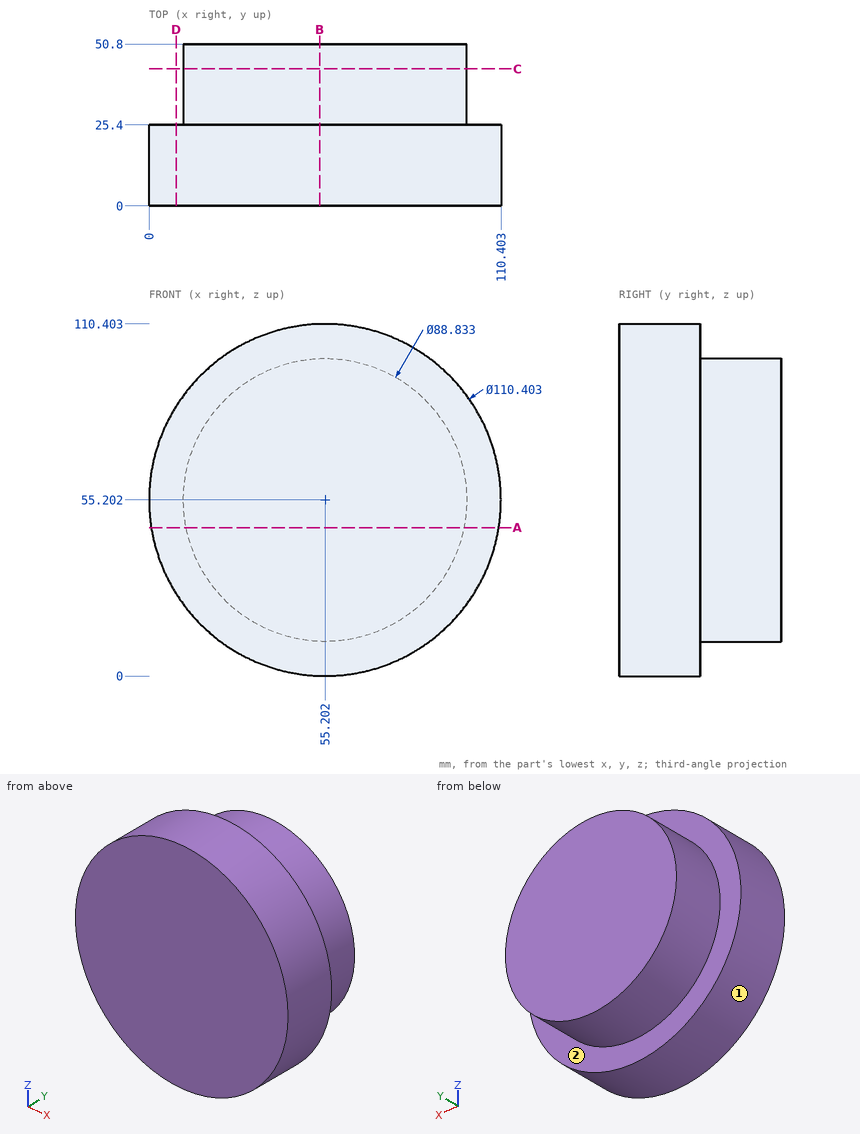
For this review, use the dimensioned drawing (mm, ordinates from the lowest corner) and the shaded views. A direction names the side the tool comes from. Round coordinates to 2 decimals unless told otherwise and drop trailing zeros. Loops run counter-clockwise (first coordinate to the right, second up) from the corner with the lowest first, then second, coordinate; pieces in that order, holes last. Notation, with made-up numbers: M 58,25 L 81,25 A34 cw 81,58 Z; hole C 19.5,83 d4. An arc over 180 degrees is marked long. Answer as CSV lines item,"result".
1. We need section D-D (x = 8.5). Give the boundary of the cut face in (y, z), plus the area to 4 significant figures.
Outcome:
outline,"M 0,25.77 L 25.4,25.77 L 25.4,84.63 L 0,84.63 Z"
area,"1,495 mm2"
2. We need section B-B (x = 53.5). Give the boundary of the cut face in (y, z) (1 decimal).
Outcome:
outline,"M 0,0 L 25.4,0 L 25.4,10.8 L 50.8,10.8 L 50.8,99.6 L 25.4,99.6 L 25.4,110.4 L 0,110.4 Z"
3. For the marked faces 1 and 2, list the 3-axis set-ups (+Z, -Z, +X, -X, +Y, -Y) from which the entire face can be reached by the end or side of a thin tool; tool diameter is ignored.
Outcome:
face 1,"+Y, -Y"
face 2,"+Y"
4. We need section C-C (y = 43). Give the boundary of the cut face in (x, z) (1 decimal).
Outcome:
outline,"C 55.2,55.2 d88.8"
5. Insertion check: pin 1 Ø10 at (y, z) = (42.5, 33) entering from +X; pin 2 Ø3 at (x, y) = (42, 13.5) entering from -Z (1 decimal); pin 3 Ø8 at (x, y) = (87, 26) entering from -Z. Each pin has a flat end and moves straight along its axis. Give the tip position at first contact, or say it passes through.
Outcome:
pin 1,"stops at x = 96.15"
pin 2,"stops at z = 1.3"
pin 3,"stops at z = 7.54"
6. We need section A-A (z = 46.5). Give the boundary of the cut face in (x, y) (1 decimal), plus the area to 3 significant figures.
Outcome:
outline,"M 0.7,0 L 109.7,0 L 109.7,25.4 L 98.8,25.4 L 98.8,50.8 L 11.6,50.8 L 11.6,25.4 L 0.7,25.4 Z"
area,"4,980 mm2"
7. To check wall thickness, follow L1, parallel to Y at x = 65, z = 6.5; L2, parallel to X at y = 21, z = 32; L3, parallel to Z at x = 26, y = 17 (1 decimal). State the ranges of each line that lie inside material, in increasing order. Write a range as [from, to].
Outcome:
L1,"y = [0, 25.4]"
L2,"x = [5.11, 105.29]"
L3,"z = [8.4, 102]"
